```python
from build123d import *

# Parameters (mm, degrees)
BOSS_EXTRUDE1_DEPTH      = 2.5
FILLET1_R                = 10
CHAMFER1_SIZE            = 1.5
M4_CLEARANCE_HOLE1_D     = 4.5
M4_CLEARANCE_HOLE1_DEPTH = 5.2
M4_CLEARANCE_HOLE1_TIP   = 1.351936393


with BuildPart() as part:
    # Sketch2 → Boss-Extrude1 (new, symmetric)
    with BuildSketch(Plane(origin=(0, 0, 0), x_dir=(1, 0, 0), z_dir=(0, 1, 0))):
        Polygon((-7.5, 26.35), (7.5, 26.35), (7.5, 7.5), (26.35, 7.5), (26.35, -7.5), (7.5, -7.5), (7.5, -26.35), (-7.5, -26.35), (-7.5, -7.5), (-26.35, -7.5), (-26.35, 7.5), (-7.5, 7.5), align=None)
    extrude(amount=BOSS_EXTRUDE1_DEPTH, both=True)

    # Fillet1
    fillet1_edges = [part.edges().sort_by_distance(p)[0] for p in [
        (7.5, 0, 7.5),
        (-7.5, 0, 7.5),
        (-7.5, 0, -7.5),
        (7.5, 0, -7.5),
    ]]
    fillet(fillet1_edges, radius=FILLET1_R)

    # Chamfer1
    chamfer1_edges = [part.edges().sort_by_distance(p)[0] for p in [
        (26.35, 0, -7.5),
        (26.35, 0, 7.5),
        (7.5, 0, 26.35),
        (-7.5, 0, 26.35),
        (-26.35, 0, 7.5),
        (-26.35, 0, -7.5),
        (-7.5, 0, -26.35),
        (7.5, 0, -26.35),
    ]]
    chamfer(chamfer1_edges, length=CHAMFER1_SIZE)

    # M4 Clearance Hole1
    with Locations(Plane(origin=(0, 2.5, 0), x_dir=(1, 0, 0), z_dir=(0, 1, 0))):
        with Locations((0, 0)):
            Hole(M4_CLEARANCE_HOLE1_D / 2, depth=M4_CLEARANCE_HOLE1_DEPTH)
            with Locations((0, 0, -(M4_CLEARANCE_HOLE1_DEPTH + M4_CLEARANCE_HOLE1_TIP / 2))):  # 118° drill point
                Cone(0, M4_CLEARANCE_HOLE1_D / 2, M4_CLEARANCE_HOLE1_TIP, mode=Mode.SUBTRACT)


solid = part.part
```
Geometry: final body of the model. Coordinates: model frame, mm. A direction names the side the tool comes from. Round coordinates to 2 decimals unless told otherwise and drop trailing zeros. Order: outer loops, then holes, each group sorted by start corner. A loop starts at its lowest first (then second) coordinate and runs counter-clockwise, first axis right, second up. Notation, with made-up numbers: M 34,54.25 L 42,54.25 A21 ccw 42,65.25 Z; hole C 68.25,64.5 d11. An arc over 180 degrees is marked long. One line per item, written item: value.
(1) Cut plane B-B (x = 0). Return the cut outline in (y, z).
Result sheet:
outline: M -2.5,-26.35 L 2.5,-26.35 L 2.5,-2.25 L -2.5,-2.25 Z; M -2.5,2.25 L 2.5,2.25 L 2.5,26.35 L -2.5,26.35 Z
(2) Cut plane C-C (y = -1.8). Return the cut outline in (x, z).
Result sheet:
outline: M -26.35,-6 L -24.85,-7.5 L -17.5,-7.5 A10 cw -7.5,-17.5 L -7.5,-24.85 L -6,-26.35 L 6,-26.35 L 7.5,-24.85 L 7.5,-17.5 A10 cw 17.5,-7.5 L 24.85,-7.5 L 26.35,-6 L 26.35,6 L 24.85,7.5 L 17.5,7.5 A10 cw 7.5,17.5 L 7.5,24.85 L 6,26.35 L -6,26.35 L -7.5,24.85 L -7.5,17.5 A10 cw -17.5,7.5 L -24.85,7.5 L -26.35,6 Z; hole C 0,0 d4.5
(3) Reachability of faces 1 (the flat face through (21, 0, 7.5)), 2 (the flat face through (-21, 0, 7.5)), 3 (the flat face through (-7.5, 0, -21)) from +Z, -Z, +X, -X, +Y, -Y: full face, straight path, thin tool, end or side. Return the list, or none.
Result sheet:
face 1: +Z, +X, +Y, -Y
face 2: +Z, -X, +Y, -Y
face 3: -Z, -X, +Y, -Y
(4) Pull-direction query (Z, two-part tool) for faces 4 (the flat face through (25.61, 0.03, -6.74)), 5 (the flat face through (-6.76, 0.03, 25.59)), 6 (the cylindrical face through (0.29, -0.03, -2.23)), 7 (the flat face through (0, 2.5, -6)); classes: pulls with the +Z half, pulls with the -Z half, needs draft (parallel to the pull), parting line crosses it, or undercut.
Result sheet:
face 4: pulls with the -Z half
face 5: pulls with the +Z half
face 6: undercut
face 7: needs draft
(5) Cut plane A-A (z = 0). Return the cut outline in (x, y), and give its area (3 significant figures).
Result sheet:
outline: M -26.35,-2.5 L -2.25,-2.5 L -2.25,2.5 L -26.35,2.5 Z; M 2.25,-2.5 L 26.35,-2.5 L 26.35,2.5 L 2.25,2.5 Z
area: 241 mm2
(6) Cut plane D-D (z = -21.5). Return the cut outline in (x, y), and give its area (3 significant figures).
Result sheet:
outline: M -7.5,-2.5 L 7.5,-2.5 L 7.5,2.5 L -7.5,2.5 Z
area: 75.0 mm2
(7) Pin query (flat end, axial travel): P1, Ø3, axis at x = 11.5, y = 1.5, coming from the -Z side; P2, Ø5, axis at x = 0, z = 0, coming from the +Y side; P3, Ø2.5, axis at x = -21, y = -0.5, coming from the -Z side. Return the tip coordinate at first contact, or that it passes through.
Result sheet:
P1: z = -10.89
P2: y = 2.5
P3: z = -7.5
(8) Line query: probe 1 along Z at (x, y) = (0, -1.15); probe 2 along X at (y, z) = (-2.2, -17); probe 3 along X at (y, z) = (-0.75, 1). Output: solid intervals per line, ascending. Write a range as [from, to].
Result sheet:
probe 1: [-26.35, -2.25], [2.25, 26.35]
probe 2: [-7.51, 7.51]
probe 3: [-26.35, -2.02], [2.02, 26.35]
